Geometry: final body of the model. Coordinates: model frame, mm. Coordinates: 2 decimals unless noted, no trailing zeros. Order: outer loops, then holes, each group sorted by start corner. A loop starts at its lowest first (then second) coordinate and runs counter-clockwise, first axis right, second up. Notation, with made-up numbers: M -32,59 L -28,59 A26 ccw -28,92 Z; hole C 37.25,88.5 d10. An arc over 180 degrees is marked long. Write item = value, one per line. Start each with the question number.
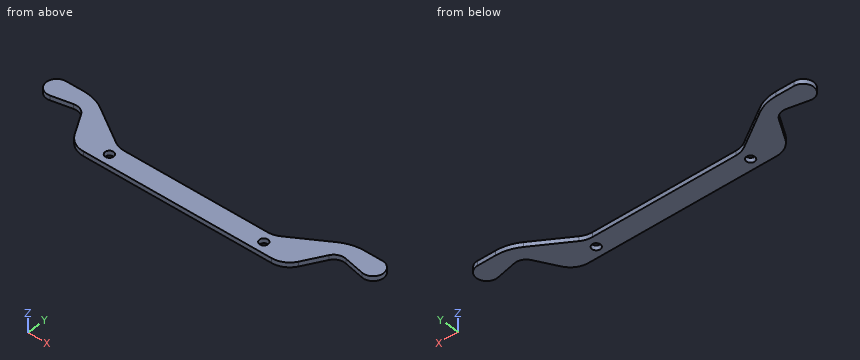
```python
from build123d import *

# Parameters (mm, degrees)
SKETCH1_R           = 2.25
BOSS_EXTRUDE1_DEPTH = 2.5


with BuildPart() as part:
    # Sketch1 → Boss-Extrude1 (new body)
    with BuildSketch(Plane.XY):
        with BuildLine():
            Line((0, 0), (-49.926715175, 0))
            ThreePointArc((-49.926715175, 0), (-55.426715175, 1.473720558), (-59.452994616, 5.5))
            Line((-59.452994616, 5.5), (-65.803847577, 16.5))
            ThreePointArc((-65.803847577, 16.5), (-68.558161164, 18.980640756), (-72.244431158, 19.369530739))
            Line((-72.244431158, 19.369530739), (-82.856553967, 17.119596823))
            ThreePointArc((-82.856553967, 17.119596823), (-89.467301609, 21.926509579), (-83.997282528, 28))
            Line((-83.997282528, 28), (-74.5, 28))
            ThreePointArc((-74.5, 28), (-68.39391207, 27.135649746), (-62.767624018, 24.61051729))
            Line((-62.767624018, 24.61051729), (-43.866187991, 12.694741355))
            ThreePointArc((-43.866187991, 12.694741355), (-41.053043965, 11.432175127), (-38, 11))
            Line((-38, 11), (0, 11))
            Line((0, 11), (0, 0))
        make_face()
        with Locations((-41, 5.5)):
            Circle(SKETCH1_R, mode=Mode.SUBTRACT)
    extrude(amount=BOSS_EXTRUDE1_DEPTH)

    # Mirror1: part across plane


with BuildPart() as part_1:
    add(part.part)
    add(part.part.mirror(Plane(origin=(0, 0, 2.5), x_dir=(0, 0, 1), z_dir=(-1, 0, 0))))


solid = part_1.part
```
Item 1: Material intervals for probe 1 along Y at (x, z) = (-4.5, 0.1); probe 2 along Y at (x, z) = (-41, 0.8); probe 3 along X at (y, z) = (25.75, 0.35), sorted ascending. Write a range as [from, to].
Item 2: Section query C-C on z = 0.8. Output: boundary loops of the cut face in (x, y), and give its area (3 significant figures).
Item 3: Section query A-A on x = 41. Output: boundary loops of the cut face in (y, z), and give its area (3 significant figures).
Item 4: First-contact query: pin 1 (1 mm diameter, centred on x = 46.5, z = 1, fed in from +Y); pin 2 (3.5 mm diameter, centred on x = -41, y = 5.5, fed in from +Z); pin 3 (1 mm diameter, centred on x = -30.5, z = 0.5, fed in from +Y); pin 4 (1.5 mm diameter, centred on y = 21.5, z = 1, fed in from +X). Flat tips, straight axial feed; report the tip coordinate or a pass-through.
Item 5: Section query B-B on y = 15. Output: boundary loops of the cut face in (x, z).
Item 6: Section query D-D on x = -32. Output: boundary loops of the cut face in (y, z), and give its area (3 significant figures).
Ans:
q1.probe_1 = [0, 11]
q1.probe_2 = [0, 3.25], [7.75, 11.42]
q1.probe_3 = [-88.43, -64.81], [64.81, 88.43]
q2.outline = M -84,28 A5.5 ccw long -82.86,17.12 L -72.24,19.37 A6 cw -65.8,16.5 L -59.45,5.5 A11 ccw -49.93,0 L 49.93,0 A11 ccw 59.45,5.5 L 65.8,16.5 A6 cw 72.24,19.37 L 82.86,17.12 A5.5 ccw long 84,28 L 74.5,28 A22 ccw 62.77,24.61 L 43.87,12.69 A11 cw 38,11 L -38,11 A11 cw -43.87,12.69 L -62.77,24.61 A22 ccw -74.5,28 Z; hole C -41,5.5 d4.5; hole C 41,5.5 d4.5
q2.area = 2,060 mm^2
q3.outline = M 0,0 L 3.25,0 L 3.25,2.5 L 0,2.5 Z; M 7.75,0 L 11.42,0 L 11.42,2.5 L 7.75,2.5 Z
q3.area = 17.3 mm^2
q4.pin_1 = 14.67
q4.pin_2 = through
q4.pin_3 = 11
q4.pin_4 = 89.49
q5.outline = M -64.94,0 L -47.52,0 L -47.52,2.5 L -64.94,2.5 Z; M 47.52,0 L 64.94,0 L 64.94,2.5 L 47.52,2.5 Z
q6.outline = M 0,0 L 11,0 L 11,2.5 L 0,2.5 Z
q6.area = 27.5 mm^2
